The figure shows three views and two pictorial views of one solid part (mm, origin at its lowest corner). Answer the questions. Coordinates: 2 decimals unless noted, no trailing zeros. Loops run counter-clockwise (first coordinate to the right, second up) from the corner with the lowest first, then second, coordinate; pieces in that order, holes last. Notation, with made-up numbers: M 66,76 L 94,76 A9 ccw 94,83 Z; hole C 84,37.25 d10. An arc over 180 degrees is marked long. Answer as a JSON object with one key per item and string values. Group by question number.
1. Straight lines are drawn through the part: L1, parallel to Z at x = 38.1, y = 5.75 (3 decimals); L2, parallel to X at y = 8.75, z = 32. For each, find the intervals that lie inside material, in ascending order.
2. A cutting plane is placed at A-A on y = 3.5. Give the vertices of the cut face in (x, z) (3 decimals).
3. Determine the mould class of the marked faces 1, 2 and 3 for opening direction Z: released by +Z, released by -Z, zero draft, split by the parting line, or undercut.
4. A cutting plane is placed at C-C on z = 38.1. Give the vertices of the cut face in (x, y) (3 decimals), and give its area (3 significant figures).
5. A cutting plane is placed at B-B on x = 38.1. Give the vertices of the cut face in (y, z) (3 decimals).
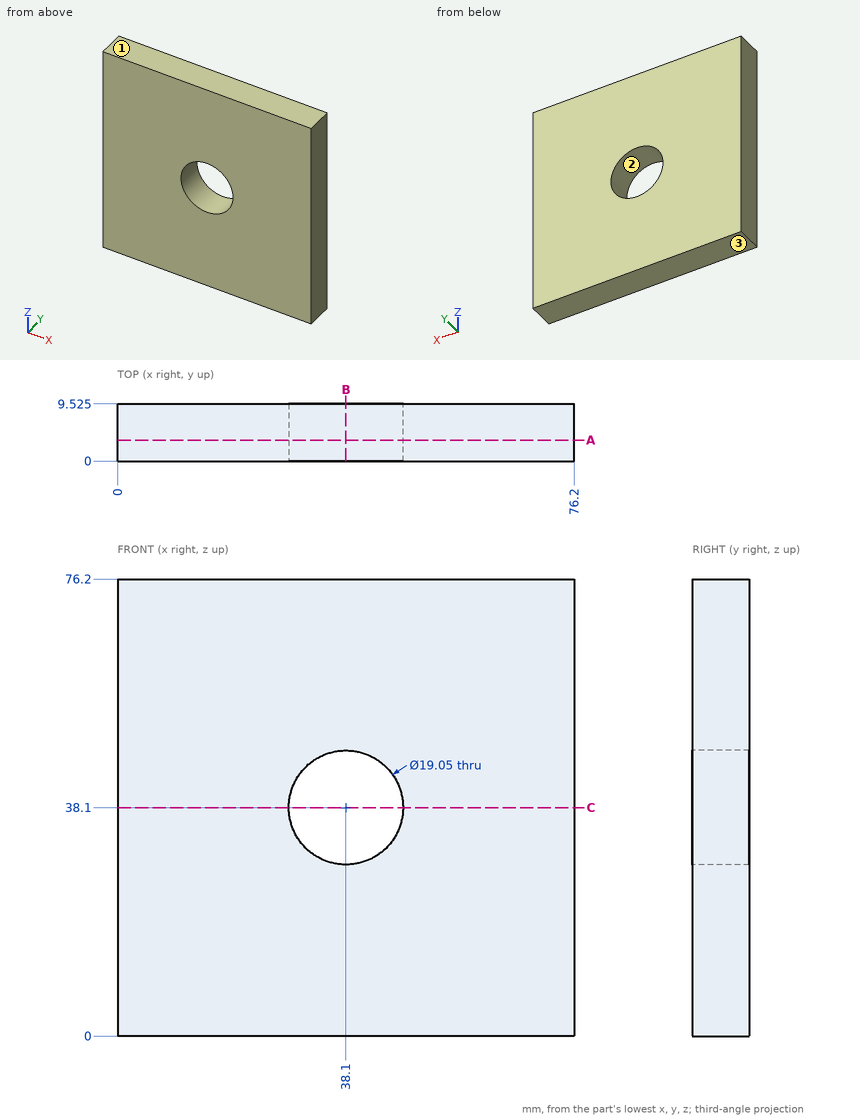
From the geometry:
{
 "1": {"L1": "z = 0 to 28.575, 47.625 to 76.2", "L2": "x = 0 to 30.78, 45.42 to 76.2"},
 "2": {"outline": "M 0,0 L 76.2,0 L 76.2,76.2 L 0,76.2 Z; hole C 38.1,38.1 d19.05"},
 "3": {"face 1": "released by +Z", "face 2": "undercut", "face 3": "released by -Z"},
 "4": {"outline": "M 0,0 L 28.575,0 L 28.575,9.525 L 0,9.525 Z; M 47.625,0 L 76.2,0 L 76.2,9.525 L 47.625,9.525 Z", "area": "544 mm²"},
 "5": {"outline": "M 0,0 L 9.525,0 L 9.525,28.575 L 0,28.575 Z; M 0,47.625 L 9.525,47.625 L 9.525,76.2 L 0,76.2 Z"}
}
